```python
from build123d import *

# Parameters (mm, degrees)
F0_R     = 1.5875
F1_DEPTH = 3.175
F2_R     = 26.9875
F2_R_2   = 26.19375
F3_DEPTH = 3.175
F5_DEPTH = 3.175


# Not quite as in the source:
# - after a boolean that leaves OpenCascade's solid faulty, fix() repairs it


with BuildPart() as f1:
    # F0 (on Top) → F1 (new body)
    with BuildSketch(Plane.XY):
        with BuildLine():
            Line((36.5125, 3.175), (29.994929259, 3.175))
            ThreePointArc((29.994929259, 3.175), (21.3281082875, 21.3281082875), (3.175, 29.994929259))
            Line((3.175, 29.994929259), (3.175, 36.5125))
            ThreePointArc((3.175, 36.5125), (0, 39.6875), (-3.175, 36.5125))
            Line((-3.175, 36.5125), (-3.175, 29.994929259))
            ThreePointArc((-3.175, 29.994929259), (-21.3281082875, 21.3281082875), (-29.994929259, 3.175))
            Line((-29.994929259, 3.175), (-30.1625, 3.175))
            Line((-30.1625, 3.175), (-36.5125, 3.175))
            ThreePointArc((-36.5125, 3.175), (-39.6875, 0), (-36.5125, -3.175))
            Line((-36.5125, -3.175), (-30.1625, -3.175))
            Line((-30.1625, -3.175), (-29.994929259, -3.175))
            ThreePointArc((-29.994929259, -3.175), (-21.3281082875, -21.3281082875), (-3.175, -29.994929259))
            Line((-3.175, -29.994929259), (-3.175, -36.5125))
            ThreePointArc((-3.175, -36.5125), (0, -39.6875), (3.175, -36.5125))
            Line((3.175, -36.5125), (3.175, -29.994929259))
            ThreePointArc((3.175, -29.994929259), (21.3281082875, -21.3281082875), (29.994929259, -3.175))
            Line((29.994929259, -3.175), (36.5125, -3.175))
            ThreePointArc((36.5125, -3.175), (39.6875, 0), (36.5125, 3.175))
        make_face()
        with Locations((0, -36.5125)):
            Circle(F0_R, mode=Mode.SUBTRACT)
        with Locations((-36.5125, 0)):
            Circle(F0_R, mode=Mode.SUBTRACT)
        with Locations((36.5125, 0)):
            Circle(F0_R, mode=Mode.SUBTRACT)
        with Locations((0, 36.5125)):
            Circle(F0_R, mode=Mode.SUBTRACT)
    extrude(amount=F1_DEPTH)

    # F2 (on face) → F3 (join)
    with BuildSketch(Plane.XY.offset(3.175)):
        Circle(F2_R)
        Circle(F2_R_2, mode=Mode.SUBTRACT)
    extrude(amount=F3_DEPTH)

    # F4 (on face) → F5 (cut)
    with BuildSketch(Plane.XY.offset(3.175)):
        with BuildLine():
            ThreePointArc((-0.8255, 26.1807388897), (-13.096875, 22.6844529204), (-22.2604349684, 13.8052734157))
            Line((-22.2604349684, 13.8052734157), (-20.1970845335, 12.6139974867))
            ThreePointArc((-20.1970845335, 12.6139974867), (-11.90625, 20.6222299276), (-0.8255, 23.7981870318))
            Line((-0.8255, 23.7981870318), (-0.8255, 26.1807388897))
        make_face()
        with BuildLine():
            ThreePointArc((0.8255, 19.0321057624), (9.525, 16.4977839421), (16.0695370777, 10.230956852))
            Line((16.0695370777, 10.230956852), (18.8213832288, 11.8197359681))
            ThreePointArc((18.8213832288, 11.8197359681), (11.1125, 19.2474145991), (0.8255, 22.2096639945))
            Line((0.8255, 22.2096639945), (0.8255, 19.0321057624))
        make_face()
        with BuildLine():
            Line((21.0225845335, -11.1841895451), (23.0859349684, -12.375465474))
            ThreePointArc((23.0859349684, -12.375465474), (25.4049183047, -6.3798640262), (26.19375, 0))
            ThreePointArc((26.19375, 0), (25.4049183047, 6.3798640262), (23.0859349684, 12.375465474))
            Line((23.0859349684, 12.375465474), (21.0225845335, 11.1841895451))
            ThreePointArc((21.0225845335, 11.1841895451), (23.8125, 0), (21.0225845335, -11.1841895451))
        make_face()
        with BuildLine():
            Line((12.7654179102, -6.4169121723), (15.5188114324, -8.0065846636))
            ThreePointArc((15.5188114324, -8.0065846636), (17.4625, 0), (15.5188114324, 8.0065846636))
            Line((15.5188114324, 8.0065846636), (12.7654179102, 6.4169121723))
            ThreePointArc((12.7654179102, 6.4169121723), (14.2875, 0), (12.7654179102, -6.4169121723))
        make_face()
        with BuildLine():
            Line((4.4747651403, -1.6303015639), (7.2495505675, -3.2323246772))
            ThreePointArc((7.2495505675, -3.2323246772), (7.9375, 0), (7.2495505675, 3.2323246772))
            Line((7.2495505675, 3.2323246772), (4.4747651403, 1.6303015639))
            ThreePointArc((4.4747651403, 1.6303015639), (4.7625, 0), (4.4747651403, -1.6303015639))
        make_face()
        with BuildLine():
            ThreePointArc((0.8255, 9.4891609086), (4.7625, 8.248891971), (7.8051044075, 5.4594844251))
            Line((7.8051044075, 5.4594844251), (10.5625136557, 7.0514753969))
            ThreePointArc((10.5625136557, 7.0514753969), (6.35, 10.9985226281), (0.8255, 12.6731428521))
            Line((0.8255, 12.6731428521), (0.8255, 9.4891609086))
        make_face()
        with BuildLine():
            ThreePointArc((-11.9399179102, 7.846720114), (-7.14375, 12.3733379566), (-0.8255, 14.2636322863))
            Line((-0.8255, 14.2636322863), (-0.8255, 17.4429772688))
            ThreePointArc((-0.8255, 17.4429772688), (-8.73125, 15.1229686136), (-14.6933114324, 9.4363926052))
            Line((-14.6933114324, 9.4363926052), (-11.9399179102, 7.846720114))
        make_face()
        with BuildLine():
            ThreePointArc((-16.8950370777, -8.8011489104), (-19.05, 0), (-16.8950370777, 8.8011489104))
            Line((-16.8950370777, 8.8011489104), (-19.6468832288, 10.3899280264))
            ThreePointArc((-19.6468832288, 10.3899280264), (-22.225, 0), (-19.6468832288, -10.3899280264))
            Line((-19.6468832288, -10.3899280264), (-16.8950370777, -8.8011489104))
        make_face()
        with BuildLine():
            ThreePointArc((-8.6306044075, -4.0296764835), (-9.525, 0), (-8.6306044075, 4.0296764835))
            Line((-8.6306044075, 4.0296764835), (-11.3880136557, 5.6216674552))
            ThreePointArc((-11.3880136557, 5.6216674552), (-12.7, 0), (-11.3880136557, -5.6216674552))
            Line((-11.3880136557, -5.6216674552), (-8.6306044075, -4.0296764835))
        make_face()
        with BuildLine():
            ThreePointArc((-0.8255, -14.2636322863), (-7.14375, -12.3733379566), (-11.9399179102, -7.846720114))
            Line((-11.9399179102, -7.846720114), (-14.6933114324, -9.4363926052))
            ThreePointArc((-14.6933114324, -9.4363926052), (-8.73125, -15.1229686136), (-0.8255, -17.4429772688))
            Line((-0.8255, -17.4429772688), (-0.8255, -14.2636322863))
        make_face()
        with BuildLine():
            ThreePointArc((-22.2604349684, -13.8052734157), (-13.096875, -22.6844529204), (-0.8255, -26.1807388897))
            Line((-0.8255, -26.1807388897), (-0.8255, -23.7981870318))
            ThreePointArc((-0.8255, -23.7981870318), (-11.90625, -20.6222299276), (-20.1970845335, -12.6139974867))
            Line((-20.1970845335, -12.6139974867), (-22.2604349684, -13.8052734157))
        make_face()
        with BuildLine():
            ThreePointArc((16.0695370777, -10.230956852), (9.525, -16.4977839421), (0.8255, -19.0321057624))
            Line((0.8255, -19.0321057624), (0.8255, -22.2096639945))
            ThreePointArc((0.8255, -22.2096639945), (11.1125, -19.2474145991), (18.8213832288, -11.8197359681))
            Line((18.8213832288, -11.8197359681), (16.0695370777, -10.230956852))
        make_face()
        with BuildLine():
            ThreePointArc((7.8051044075, -5.4594844251), (4.7625, -8.248891971), (0.8255, -9.4891609086))
            Line((0.8255, -9.4891609086), (0.8255, -12.6731428521))
            ThreePointArc((0.8255, -12.6731428521), (6.35, -10.9985226281), (10.5625136557, -7.0514753969))
            Line((10.5625136557, -7.0514753969), (7.8051044075, -5.4594844251))
        make_face()
        with BuildLine():
            ThreePointArc((-0.8255, -4.6904110694), (-2.38125, -4.1244459855), (-3.6492651403, -3.0601095055))
            Line((-3.6492651403, -3.0601095055), (-6.4240505675, -4.6621326189))
            ThreePointArc((-6.4240505675, -4.6621326189), (-3.96875, -6.8740766425), (-0.8255, -7.8944572961))
            Line((-0.8255, -7.8944572961), (-0.8255, -4.6904110694))
        make_face()
        with BuildLine():
            ThreePointArc((-3.6492651403, 3.0601095055), (-2.38125, 4.1244459855), (-0.8255, 4.6904110694))
            Line((-0.8255, 4.6904110694), (-0.8255, 7.8944572961))
            ThreePointArc((-0.8255, 7.8944572961), (-3.96875, 6.8740766425), (-6.4240505675, 4.6621326189))
            Line((-6.4240505675, 4.6621326189), (-3.6492651403, 3.0601095055))
        make_face()
        with BuildLine():
            Line((0.8255, 1.4298079416), (2.2423170542, 2.2478076493))
            ThreePointArc((2.2423170542, 2.2478076493), (1.5875, 2.749630657), (0.8255, 3.065807357))
            Line((0.8255, 3.065807357), (0.8255, 1.4298079416))
        make_face()
        with BuildLine():
            Line((0.8255, -1.4298079416), (0.8255, -3.065807357))
            ThreePointArc((0.8255, -3.065807357), (1.5875, -2.749630657), (2.2423170542, -2.2478076493))
            Line((2.2423170542, -2.2478076493), (0.8255, -1.4298079416))
        make_face()
        with BuildLine():
            Line((-1.651, 0), (-3.0678170542, 0.8179997077))
            ThreePointArc((-3.0678170542, 0.8179997077), (-3.175, 0), (-3.0678170542, -0.8179997077))
            Line((-3.0678170542, -0.8179997077), (-1.651, 0))
        make_face()
    extrude(amount=-F5_DEPTH, mode=Mode.SUBTRACT)

    add(f1.part.fix(), mode=Mode.REPLACE)


solid = f1.part
```
Source: CAD feature listing. Evaluate the final solid. Frame: model axes, mm. A direction names the side the tool comes from. Round coordinates to 2 decimals unless told otherwise and drop trailing zeros. Loops run counter-clockwise (first coordinate to the right, second up) from the corner with the lowest first, then second, coordinate; pieces in that order, holes last. Notation, with made-up numbers: M -16.5,-18 L -4.5,-18 A17 cw -4.5,5 Z; hole C 16,13 d6. An arc over 180 degrees is marked long. Use a Markdown table: item, result. Add a question column.
1. Set-up query: faces 3 (the flat face through (-0.826, -6, 2)), 4 (the flat face through (-1.5, 0.4, 3.175)). Return all of +Z, -Z, +X, -X, +Y, -Y with unobstructed straight access to the full face (end or side cutting, diameter ignored); none if empty.
2. Ray query, line 1 along Y through (x, z) = (0, 1.3) (1 decimal); line 2 along X through (y, z) = (1, 4.25); line 3 along Y through (x, z) = (0, 3.5). Return the intervals inside material, ascending. Write a range as [from, to].
3. Pull-direction query (Y, two-part tool) for faces 1 (the cylindrical face through (-9.525, -0.058, 1.61)), 2 (the flat face through (17.4, 11, 1.6)); classes: +Y half, -Y half, draft (parallel to the pull), parting line (faces both ways), or undercut.
4. Contact query for flat-ended pins moving along their axis: pin 1 (2.5 mm diameter, centred on x = 0, y = 36.51, fed in from -Z); pin 2 (1.6 mm diameter, centred on y = -20.5, z = 2, fed in from +X); pin 3 (1.6 mm diameter, centred on y = -34, z = 2, fed in from -X) (3 decimals); pin 4 (2.5 mm diameter, centred on y = 11, z = 2, fed in from +X). Output: stop coordinate, or through.
5. Cut plane A-A, the plane z = 1.75. State how many separate pieces and enclosed holes the cut face has, and give its area (3 significant figures).
6. Cut plane B-B, the plane y = 31. Output: boundary loops of the cut face in (x, z) (3 decimals).
Solution:
| question | item | result |
|---|---|---|
| 1 | face 3 | +Z, -Z |
| 1 | face 4 | +Z |
| 2 | line 1 | y = [-39.7, -38.1], [-34.9, 34.9], [38.1, 39.7] |
| 2 | line 2 | x = [-26.97, -26.17], [26.17, 26.97] |
| 2 | line 3 | y = [-26.99, -26.19], [26.19, 26.99] |
| 3 | face 1 | undercut |
| 3 | face 2 | undercut |
| 4 | pin 1 | passes through |
| 4 | pin 2 | stops at x = 22.84 |
| 4 | pin 3 | stops at x = -3.175 |
| 4 | pin 4 | stops at x = 28.54 |
| 5 | separate pieces | 1 |
| 5 | enclosed holes | 22 |
| 5 | area | 2,400 mm2 |
| 6 | outline | M -3.175,0 L 3.175,0 L 3.175,3.175 L -3.175,3.175 Z |
